Input: part model. Units: mm. Frame: model coordinates. A direction names the side the tool comes from. Coordinates: 2 decimals unless noted, no trailing zeros. Order: outer loops, then holes, each group sorted by start corner. A loop starts at its lowest first (then second) coordinate and runs counter-clockwise, first axis right, second up. Notation, with made-up numbers: (37.25, -28.75) - (85.25, -28.75) arc R13 ccw to (85.25, -8.75) - close; hole circle Ø7 at (79.25, 59.5). An arc over 180 degrees is marked (long way). Answer as CSV lines item,"result". Start each with the question number.
Item 1: Material intervals for line 1 along X through (y, z) = (14, 0.35); line 2 along Y through (x, z) = (36.5, 2); line 3 along Y through (x, z) = (43.5, 1.3), sorted ascending.
Item 2: First-contact query: pin 1 (1 mm diameter, centred on y = -1.5, z = 2, fed in from +X); pin 2 (1.5 mm diameter, centred on y = 6, z = 2.5, fed in from -X); pin 3 (0.9 mm diameter, centred on x = 19, z = 2, fed in from -Y); pin 4 (4 mm diameter, centred on x = 38, y = 8, fed in from -Z). Flat tips, straight axial feed; report the tip coordinate or a pass-through.
Item 3: Section A-A (x = 43.5). Output: boundary loops of the cut face in (y, z).
Item 4: Draft query along Y for faces 4 (the flat face through (41, 9, 1)), 5 (the flat face through (82, 15, 1)), 6 (the flat face through (55, 1, 1)), 7 (the flat face through (40, 0, 1)). Return one class per face: +Y half, -Y half, draft (parallel to the pull), parting line (faces both ways), or undercut.
Item 5: Section D-D (x = 24.5). Output: boundary loops of the cut face in (y, z), and give its area (3 significant figures).
Item 6: Section B-B (y = 11). Output: boundary loops of the cut face in (x, z), and give its area (3 significant figures).
Item 7: Section C-C (x = 67.5). Output: boundary loops of the cut face in (y, z), and give its area (3 significant figures).
Item 8: Access query for faces 1 (the flat face through (80, 0, 1)), 2 (the flat face through (35, 3, 1)), 3 (the flat face through (0, 2, 1)). Directions: +Z, -Z, +X, -X, +Y, -Y. A direction counts if a zero-diameter tool reaches every point of the face in a straight line with its end or side. Return the directions, or none.
from build123d import *

# Parameters (mm, degrees)
BOSS_EXTRUDE1_DEPTH = 3
FILLET1_R           = 0.5


with BuildPart() as part:
    # Sketch1 → Boss-Extrude1 (new body)
    with BuildSketch(Plane.XY):
        Polygon((0, 0), (30, 0), (30, -3), (45, -3), (45, 0), (35, 0), (35, 1), (75, 1), (75, 0), (85, 0), (85, 15), (79, 15), (79, 3), (66, 3), (66, 15), (60, 15), (60, 3), (47, 3), (47, 15), (41, 15), (41, 3), (28, 3), (28, 15), (22, 15), (22, 3), (0, 3), align=None)
    extrude(amount=BOSS_EXTRUDE1_DEPTH)

    # Fillet1
    fillet1_edges = [part.edges().sort_by_distance(p)[0] for p in [
        (22, 3, 1.5),
        (22, 15, 1.5),
        (28, 15, 1.5),
        (28, 3, 1.5),
        (41, 3, 1.5),
        (47, 15, 1.5),
        (47, 3, 1.5),
        (66, 3, 1.5),
        (60, 3, 1.5),
        (60, 15, 1.5),
        (66, 15, 1.5),
        (79, 3, 1.5),
        (79, 15, 1.5),
        (85, 15, 1.5),
        (85, 0, 1.5),
        (75, 1, 1.5),
        (75, 0, 1.5),
        (0, 3, 1.5),
        (0, 0, 1.5),
        (30, 0, 1.5),
        (30, -3, 1.5),
        (45, -3, 1.5),
        (45, 0, 1.5),
        (35, 0, 1.5),
        (35, 1, 1.5),
    ]]
    fillet(fillet1_edges, radius=FILLET1_R - 0.0001)  # a hair under: the kernel refuses the full size


solid = part.part
Determined:
1,line 1,"x = 22 to 28, 41 to 47, 60 to 66, 79 to 85"
1,line 2,"y = -3 to 0, 1 to 3"
1,line 3,"y = -3 to 0, 1 to 15"
2,pin 1,"stops at x = 45"
2,pin 2,"stops at x = 22"
2,pin 3,"stops at y = 0"
2,pin 4,"passes through"
3,outline,"(-3, 0) - (0, 0) - (0, 3) - (-3, 3) - close; (1, 0) - (15, 0) - (15, 3) - (1, 3) - close"
4,face 4,"draft"
4,face 5,"+Y half"
4,face 6,"undercut"
4,face 7,"undercut"
5,outline,"(0, 0) - (15, 0) - (15, 3) - (0, 3) - close"
5,area,"45.0 mm^2"
6,outline,"(22, 0) - (28, 0) - (28, 3) - (22, 3) - close; (41, 0) - (47, 0) - (47, 3) - (41, 3) - close; (60, 0) - (66, 0) - (66, 3) - (60, 3) - close; (79, 0) - (85, 0) - (85, 3) - (79, 3) - close"
6,area,"72.0 mm^2"
7,outline,"(1, 0) - (3, 0) - (3, 3) - (1, 3) - close"
7,area,"6.00 mm^2"
8,face 1,"+Z, -Z, +X, -Y"
8,face 2,"+Z, -Z, +Y"
8,face 3,"+Z, -Z, -X, +Y, -Y"
